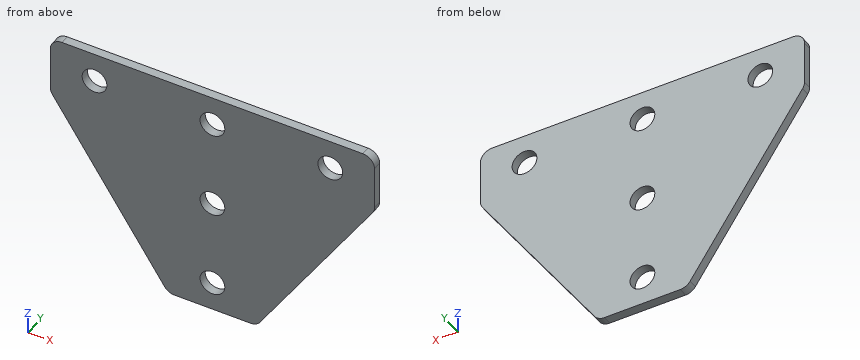
```python
from build123d import *

# Parameters (mm, degrees)
SKETCH_1_R      = 2.1
EXTRUDE_1_DEPTH = 1.5
FILLET_1_R      = 2


with BuildPart() as part:
    # ｽｹｯﾁ1 → ﾎﾞｽ - 押し出し1 (new body)
    with BuildSketch(Plane(origin=(0, 0, 0), x_dir=(1, 0, 0), z_dir=(0, 1, 0))):
        Polygon((0, 0), (55, 0), (55, 10), (35, 40), (20, 40), (0, 10), align=None)
        with Locations(Location((7.5, 5, 0), (0, 0, 270))):
            Circle(SKETCH_1_R, mode=Mode.SUBTRACT)
        with Locations(Location((47.5, 5, 0), (0, 0, 90))):
            Circle(SKETCH_1_R, mode=Mode.SUBTRACT)
        with Locations(Location((27.5, 5, 0), (0, 0, 270))):
            Circle(SKETCH_1_R, mode=Mode.SUBTRACT)
        with Locations(Location((27.5, 35, 0), (0, 0, 270))):
            Circle(SKETCH_1_R, mode=Mode.SUBTRACT)
        with Locations(Location((27.5, 20, 0), (0, 0, 270))):
            Circle(SKETCH_1_R, mode=Mode.SUBTRACT)
    extrude(amount=EXTRUDE_1_DEPTH)

    # ﾌｨﾚｯﾄ1
    fillet_1_edges = [part.edges().sort_by_distance(p)[0] for p in [
        (0, 0.75, -10),
        (20, 0.75, -40),
        (35, 0.75, -40),
        (55, 0.75, -10),
        (55, 0.75, 0),
        (0, 0.75, 0),
    ]]
    fillet(fillet_1_edges, radius=FILLET_1_R)


solid = part.part
```
CAD build for the part. Positions are in the model's coordinates, mm. Coordinates: 2 decimals unless noted, no trailing zeros. Write each loop counter-clockwise with the first axis right and the second up, starting at its lowest first coordinate (ties: lowest second). Pieces come first, ordered by that corner, then holes. Notation, with made-up numbers: (-28, -10) -> (25, -10) arc R21 ccw to (25, 15) -> close; hole circle Ø8 at (37, 37.25). An arc over 180 degrees is marked (long way). Return JSON: item names as keys, results as strings. Group by question number.
Q1. Cut at C-C, the plane z = -5. Give the cut face in (x, y).
Q2. Cut at B-B, the plane y = 0.7. Give the cut face in (x, z), then the cut area to 3 significant figures.
Q3. Cut at A-A, the plane x = 27.5. Give the cut face in (y, z).
Q4. Cut at D-D, the plane x = 7.5. Give the cut face in (y, z).
Q5. Drill centre lines: line 1 (X direction, y = 0.75, z = -5); line 2 (X direction, y = 0.45, z = -20); line 3 (Z direction, x = 47.5, y = 1.15). Where is each one in solid material? Low to high.
Returned:
{
 "1": {"outline": "(0, 0) -> (5.4, 0) -> (5.4, 1.5) -> (0, 1.5) -> close; (9.6, 0) -> (25.4, 0) -> (25.4, 1.5) -> (9.6, 1.5) -> close; (29.6, 0) -> (45.4, 0) -> (45.4, 1.5) -> (29.6, 1.5) -> close; (49.6, 0) -> (55, 0) -> (55, 1.5) -> (49.6, 1.5) -> close"},
 "2": {"outline": "(0, -9.39) arc R2 ccw to (0.34, -10.5) -> (19.41, -39.11) arc R2 ccw to (21.07, -40) -> (33.93, -40) arc R2 ccw to (35.59, -39.11) -> (54.66, -10.5) arc R2 ccw to (55, -9.39) -> (55, -2) arc R2 ccw to (53, 0) -> (2, 0) arc R2 ccw to (0, -2) -> close; hole circle Ø4.2 at (7.5, -5); hole circle Ø4.2 at (27.5, -35); hole circle Ø4.2 at (27.5, -20); hole circle Ø4.2 at (27.5, -5); hole circle Ø4.2 at (47.5, -5)", "area": "1,530 mm2"},
 "3": {"outline": "(0, -40) -> (1.5, -40) -> (1.5, -37.1) -> (0, -37.1) -> close; (0, -32.9) -> (1.5, -32.9) -> (1.5, -22.1) -> (0, -22.1) -> close; (0, -17.9) -> (1.5, -17.9) -> (1.5, -7.1) -> (0, -7.1) -> close; (0, -2.9) -> (1.5, -2.9) -> (1.5, 0) -> (0, 0) -> close"},
 "4": {"outline": "(0, -21.25) -> (1.5, -21.25) -> (1.5, -7.1) -> (0, -7.1) -> close; (0, -2.9) -> (1.5, -2.9) -> (1.5, 0) -> (0, 0) -> close"},
 "5": {"line 1": "x = 0 to 5.4, 9.6 to 25.4, 29.6 to 45.4, 49.6 to 55", "line 2": "x = 6.67 to 25.4, 29.6 to 48.33", "line 3": "z = -21.25 to -7.1, -2.9 to 0"}
}
